Geometry: final body of the model. Coordinates: model frame, mm. Face numbers are marked on the shaded views. A direction names the side the tool comes from. Give positions to 0.01 mm unless a question says otherwise; leave off trailing zeros. Loops run counter-clockwise (first coordinate to the right, second up) from the corner with the lowest first, then second, coordinate; pieces in that order, holes last.
1. Section B-B, the plane y = -35. Output: boundary loops of the cut face in (x, z).
2. Section C-C, the plane x = 34.5. Output: boundary loops of the cut face in (y, z), then the cut area to 3 significant figures.
3. Access query for the marked faces 1, 2 and 3. Directions: +Z, -Z, +X, -X, +Y, -Y. A direction counts if a zero-diameter tool reaches every point of the face in a straight line with its end or side. Return the directions, or none.
4. Section A-A, the plane z = -6. Output: boundary loops of the cut face in (x, y).
5. Material intervals for line 1 along X through (y, z) = (-40, -10.75); line 2 along X through (y, z) = (7.35, -6); line 3 along X through (y, z) = (-5, -12), sorted ascending.
6. First-contact query: P1, Ø4.5, axis at x = 18, z = -5, coming from the +Y side; P2, Ø3, axis at x = 2.5, z = -7, coming from the +Y side; P3, Ø5, axis at y = -10, z = -8.5, coming from the -X side. Flat tips, straight axial feed; report the tip coordinate or a pass-through.
7. Section D-D, the plane y = 1.5. Output: boundary loops of the cut face in (x, z), then the cut area to 4 significant figures.
8. Draft query along Y for the marked faces 4, 5, 6 and 7. Return one class per face: +Y half, -Y half, draft (parallel to the pull), parting line (faces both ways), or undercut.
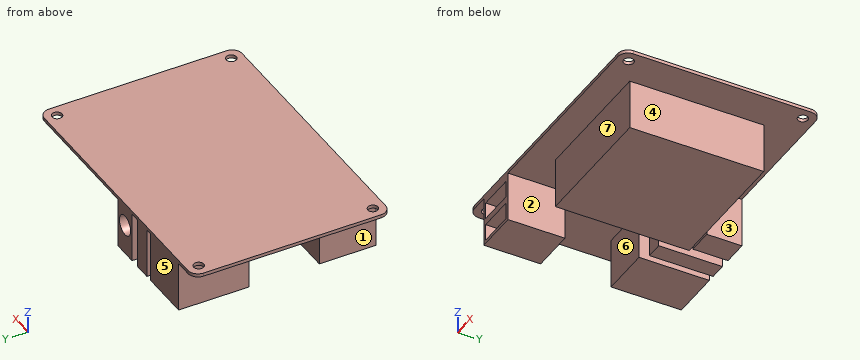
from build123d import *

# Parameters (mm, degrees)
SKETCH1_W           = 83
SKETCH1_H           = 59
SKETCH1_R           = 1.5
BOSS_EXTRUDE1_DEPTH = 1
SKETCH2_W           = 15
SKETCH2_H           = 21
SKETCH2_W_2         = 13
SKETCH2_H_2         = 17
SKETCH2_W_3         = 5
SKETCH2_H_3         = 19
SKETCH2_W_4         = 7.5
SKETCH2_H_4         = 10.5
SKETCH2_W_5         = 40
SKETCH2_H_5         = 40
BOSS_EXTRUDE2_DEPTH = 15
SKETCH3_R           = 3
CUT_EXTRUDE1_DEPTH  = 5
SKETCH4_W           = 11
SKETCH4_H           = 5
CUT_EXTRUDE2_DEPTH  = 10
FILLET1_R           = 3


with BuildPart() as part:
    # Sketch1 → Boss-Extrude1 (new body)
    with BuildSketch(Plane.XY):
        with Locations((6.725862069, -19.339655172)):
            Rectangle(SKETCH1_W, SKETCH1_H)
        with Locations((-31.274137931, 6.660344828)):
            Circle(SKETCH1_R, mode=Mode.SUBTRACT)
        with Locations((44.725862069, 6.660344828)):
            Circle(SKETCH1_R, mode=Mode.SUBTRACT)
        with Locations((44.725862069, -45.339655172)):
            Circle(SKETCH1_R, mode=Mode.SUBTRACT)
        with Locations((-31.274137931, -45.339655172)):
            Circle(SKETCH1_R, mode=Mode.SUBTRACT)
    extrude(amount=BOSS_EXTRUDE1_DEPTH)

    # Sketch2 → Boss-Extrude2 (add)
    with BuildSketch(Plane(origin=(0, 0, 0), x_dir=(-1, 0, 0), z_dir=(0, 0, -1))):
        with Locations((19.274137931, -0.339655172)):
            Rectangle(SKETCH2_W, SKETCH2_H)
        with Locations((20.274137931, -40.339655172)):
            Rectangle(SKETCH2_W_2, SKETCH2_H_2)
        with Locations((7.274137931, 0.660344828)):
            Rectangle(SKETCH2_W_3, SKETCH2_H_3)
        with Locations((-1.975862069, 4.910344828)):
            Rectangle(SKETCH2_W_4, SKETCH2_H_4)
        with Locations((-17.225862069, -20.839655172)):
            Rectangle(SKETCH2_W_5, SKETCH2_H_5)
    extrude(amount=BOSS_EXTRUDE2_DEPTH)

    # Sketch3 → Cut-Extrude1 (cut)
    with BuildSketch(Plane(origin=(0, 10.160344828, 0), x_dir=(1, 0, 0), z_dir=(0, 1, 0))):
        with Locations(Location((1.975862069, 6, 0), (0, 0, 270))):
            Circle(SKETCH3_R)
    extrude(amount=-CUT_EXTRUDE1_DEPTH, mode=Mode.SUBTRACT)

    # Sketch4 → Cut-Extrude2 (cut)
    with BuildSketch(Plane.XZ.offset(48.839655172)):
        with Locations((-20.274137931, -4.5)):
            Rectangle(SKETCH4_W, SKETCH4_H)
        with Locations((-20.274137931, -11.5)):
            Rectangle(SKETCH4_W, SKETCH4_H)
    extrude(amount=-CUT_EXTRUDE2_DEPTH, mode=Mode.SUBTRACT)

    # Fillet1
    fillet1_edges = [part.edges().sort_by_distance(p)[0] for p in [
        (48.225862069, -48.839655172, 0.5),
        (-34.774137931, -48.839655172, 0.5),
        (-34.774137931, 10.160344828, 0.5),
        (48.225862069, 10.160344828, 0.5),
    ]]
    fillet(fillet1_edges, radius=FILLET1_R)


solid = part.part
Answers below:
1. outline: (-34.77, 0) - (-26.77, 0) - (-26.77, -15) - (-13.77, -15) - (-13.77, 0) - (-2.77, 0) - (-2.77, -15) - (37.23, -15) - (37.23, 0) - (48.23, 0) - (48.23, 1) - (-34.77, 1) - close
2. outline: (-48.84, 0) - (-40.84, 0) - (-40.84, -15) - (-0.84, -15) - (-0.84, 0) - (10.16, 0) - (10.16, 1) - (-48.84, 1) - close
2. area: 659 mm2
3. face 1: -Z, -X, +Y, -Y
3. face 2: -Z, -Y
3. face 3: -Z, +X, +Y
4. outline: (-26.77, -48.84) - (-25.77, -48.84) - (-25.77, -38.84) - (-14.77, -38.84) - (-14.77, -48.84) - (-13.77, -48.84) - (-13.77, -31.84) - (-26.77, -31.84) - close; (-26.77, -10.84) - (-11.77, -10.84) - (-11.77, 10.16) - (-26.77, 10.16) - close; (-9.77, -8.84) - (-4.77, -8.84) - (-4.77, 10.16) - (-9.77, 10.16) - close; (-2.77, -40.84) - (37.23, -40.84) - (37.23, -0.84) - (-2.77, -0.84) - close; (-1.77, -0.34) - (5.73, -0.34) - (5.73, 10.16) - (4.98, 10.16) - (4.98, 5.16) - (-1.02, 5.16) - (-1.02, 10.16) - (-1.77, 10.16) - close
5. line 1: x = -26.77 to -25.77, -14.77 to -13.77, -2.77 to 37.23
5. line 2: x = -26.77 to -11.77, -9.77 to -4.77, -1.77 to -1.02, 4.98 to 5.73
5. line 3: x = -26.77 to -11.77, -9.77 to -4.77, -2.77 to 37.23
6. P1: stops at y = -0.84
6. P2: stops at y = 5.16
6. P3: stops at x = -26.77
7. outline: (-34.77, 0) - (-26.77, 0) - (-26.77, -15) - (-11.77, -15) - (-11.77, 0) - (-9.77, 0) - (-9.77, -15) - (-4.77, -15) - (-4.77, 0) - (-1.77, 0) - (-1.77, -15) - (5.73, -15) - (5.73, 0) - (48.23, 0) - (48.23, 1) - (-34.77, 1) - close
7. area: 495.5 mm2
8. face 4: draft
8. face 5: +Y half
8. face 6: undercut
8. face 7: -Y half
